Source: CAD feature listing. Evaluate the final solid. Frame: model axes, mm. Face numbers are marked on the shaded views. A direction names the side the tool comes from. Round coordinates to 2 decimals unless told otherwise and drop trailing zeros. Loops run counter-clockwise (first coordinate to the right, second up) from the corner with the lowest first, then second, coordinate; pieces in that order, holes last. Notation, with made-up numbers: M 75.25,39.5 L 110.25,39.5 A6 ccw 110.25,47.5 Z; hole C 81,84.5 d3. An arc over 180 degrees is marked long. Answer as a JSON object with one key per item and string values.
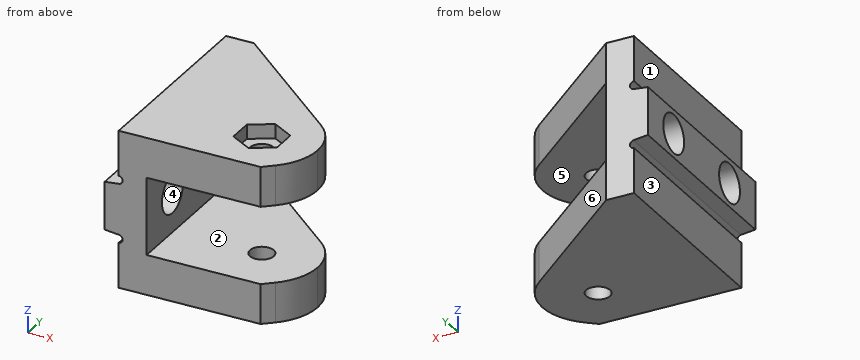
from build123d import *

# Parameters (mm, degrees)
F0_W          = 18
F0_H          = 5
F1_DEPTH      = 25
F2_R          = 1.5
F3_DEPTH      = 14.691
F3_DEPTH_BACK = 25
F0_W_2        = 8
F0_H_2        = 0.52
F5_DEPTH      = 25
F6_R          = 2.425
F7_DEPTH      = 25
F8_R          = 1.5
F9_DEPTH      = 1.8


with BuildPart() as f1:
    # F0 (on Front) → F1 (new body)
    with BuildSketch(Plane.XZ):
        with BuildLine():
            Line((2, -9.845), (5.5, -9.845))
            Line((5.5, -9.845), (5.5, -4.845))
            Line((5.5, -4.845), (5.5, 4.845))
            Line((5.5, 4.845), (5.5, 9.845))
            Line((5.5, 9.845), (2, 9.845))
            Line((2, 9.845), (2, 4.196959))
            ThreePointArc((2, 4.196959), (2.499239, 3.724532), (2.055063, 3.2))
            Line((2.055063, 3.2), (0.25, 3))
            Line((0.25, 3), (0.25, -3))
            Line((0.25, -3), (2.055063, -3.2))
            ThreePointArc((2.055063, -3.2), (2.499239, -3.724532), (2, -4.196959))
            Line((2, -4.196959), (2, -9.845))
        make_face()
        with Locations((14.5, -7.345)):
            Rectangle(F0_W, F0_H)
        with Locations((14.5, 7.345)):
            Rectangle(F0_W, F0_H)
    extrude(amount=F1_DEPTH)

    # F2 (on face) → F3 (cut, two sides)
    with BuildSketch(Plane(origin=(0, 0, 4.845), x_dir=(1, 0, 0), z_dir=(0, 0, -1))) as f3_sk:
        with BuildLine():
            Line((23.5, 25), (19.784899, 25))
            Line((19.784899, 25), (21.046038, 23.922926))
            ThreePointArc((21.046038, 23.922926), (22.856975, 21.530677), (23.5, 18.6))
            Line((23.5, 18.6), (23.5, 25))
        make_face()
        with BuildLine():
            Line((23.5, 0), (23.5, 18.6))
            ThreePointArc((23.5, 18.6), (22.856975, 15.669323), (21.046038, 13.277074))
            Line((21.046038, 13.277074), (5.5, 0))
            Line((5.5, 0), (23.5, 0))
        make_face()
        with Locations((16.5, 18.6)):
            Circle(F2_R)
    extrude(amount=F3_DEPTH, mode=Mode.SUBTRACT)
    extrude(f3_sk.sketch, amount=-F3_DEPTH_BACK, mode=Mode.SUBTRACT)

    # F0 (on Front) → F5 (cut)
    with BuildSketch(Plane.XZ):
        Polygon((10.765, 4.225), (10.765, -4.225), (12.5, -4.225), (20.5, -4.225), (22.235, -4.225), (22.235, 4.225), (20.5, 4.225), (12.5, 4.225), align=None)
        with Locations((16.5, 4.485)):
            Rectangle(F0_W_2, F0_H_2)
        with Locations((16.5, -4.485)):
            Rectangle(F0_W_2, F0_H_2)
    extrude(amount=F5_DEPTH, mode=Mode.SUBTRACT)

    # F6 (on face) → F7 (cut)
    with BuildSketch(Plane.YZ.offset(5.5)):
        with Locations((-6, 0)):
            Circle(F6_R)
        with Locations((-19, 0)):
            Circle(F6_R)
    extrude(amount=-F7_DEPTH, mode=Mode.SUBTRACT)

    # F8 (on face) → F9 (cut)
    with BuildSketch(Plane.XY.offset(9.845)):
        Polygon((19.225, -20.173279), (19.225, -17.026721), (16.5, -15.453441), (13.775, -17.026721), (13.775, -20.173279), (16.5, -21.746559), align=None)
        with Locations((16.5, -18.6)):
            Circle(F8_R, mode=Mode.SUBTRACT)
    extrude(amount=-F9_DEPTH, mode=Mode.SUBTRACT)


solid = f1.part
Item 1: Line query: probe 1 along Z at (x, y) = (11, -14) (3 decimals); probe 2 along X at (y, z) = (-18.6, 6.55); probe 3 along Z at (x, y) = (15, -19.25) (3 decimals). Output: solid intervals per line, ascending. Write a range as from..to.
Answer sheet:
{"probe 1": "z = -9.845..-4.845, 4.845..9.845", "probe 2": "x = 2..15, 18..23.5", "probe 3": "z = -9.845..-4.845, 4.845..8.045"}
Item 2: Section C-C on z = -8.25. Return the cut outline in (x, y), then the cut area to 3 significant figures.
Answer sheet:
{"outline": "M 2,-25 L 19.78,-25 L 21.05,-23.92 A7 ccw 23.5,-18.6 A7 ccw 21.05,-13.28 L 5.5,0 L 2,0 Z; hole C 16.5,-18.6 d3", "area": "383 mm²"}
Item 3: Section B-B on y = -17.5. Give the number of separate pieces and of enclosed holes in the cut face, then the cut area to 3 significant figures.
Answer sheet:
{"separate pieces": "4", "enclosed holes": "0", "area": "212 mm²"}
Item 4: Pull-direction query (Y, two-part tool) for the marked faces 4, 5 and 6; classes: pulls with the +Y half, pulls with the -Y half, needs draft (parallel to the pull), parting line crosses it, or undercut.
Answer sheet:
{"face 4": "undercut", "face 5": "needs draft", "face 6": "pulls with the +Y half"}
Item 5: Contact query for flat-ended pins moving along their axis: pin 1 Ø4 at (y, z) = (-6, 0) entering from -X; pin 2 Ø3 at (y, z) = (-14.5, 5.5) entering from -X; pin 3 Ø2.5 at (x, y) = (16.5, -17) entering from +Z (3 decimals). Output: stop coordinate, or through.
Answer sheet:
{"pin 1": "passes through", "pin 2": "stops at x = 2", "pin 3": "stops at z = 8.045"}
Item 6: Section A-A on z = 0. Return the cut outline in (x, y) (3 decimals).
Answer sheet:
{"outline": "M 0.25,-25 L 5.5,-25 L 5.5,-21.425 L 0.25,-21.425 Z; M 0.25,-16.575 L 5.5,-16.575 L 5.5,-8.425 L 0.25,-8.425 Z; M 0.25,-3.575 L 5.5,-3.575 L 5.5,0 L 0.25,0 Z"}
Item 7: Section D-D on x = 10.5. Return the cut outline in (y, z) (3 decimals).
Answer sheet:
{"outline": "M -25,-9.845 L -4.27,-9.845 L -4.27,-4.845 L -25,-4.845 Z; M -25,4.845 L -4.27,4.845 L -4.27,9.845 L -25,9.845 Z"}
Item 8: Access query for the marked faces 1, 2 and 3. Directions: +Z, -Z, +X, -X, +Y, -Y. A direction counts if a zero-diameter tool reaches every point of the face in a straight line with its end or side. Return the directions, or none.
Answer sheet:
{"face 1": "+Z, -X, +Y, -Y", "face 2": "+X, +Y, -Y", "face 3": "-Z, -X, +Y, -Y"}
